Build history of the part. All positions in model axes, mm. A direction names the side the tool comes from. Round coordinates to 2 decimals unless told otherwise and drop trailing zeros. Loops run counter-clockwise (first coordinate to the right, second up) from the corner with the lowest first, then second, coordinate; pieces in that order, holes last. Notation, with made-up numbers: M -39,-31 L 2,-31 A34 ccw 2,1 Z; hole C -30.5,10.5 d10. An arc over 180 degrees is marked long. Use one line per item in the form item = value. Start each with the question number.
```python
from build123d import *

# Parameters (mm, degrees)
F1_DEPTH = 70
F2_T     = -1
F4_DEPTH = 4


with BuildPart() as f1:
    # F0 (on Top) → F1 (new body)
    with BuildSketch(Plane.XY):
        Polygon((50.477442, 204.086703), (-26.674857, 204.086703), (-79.522558, -15.913297), (-79.522558, -65.913297), (50.477442, -65.913297), align=None)
    extrude(amount=F1_DEPTH)

    # F2
    f2_openings = [f1.faces().sort_by_distance(p)[0] for p in [
        (-5.117094, 56.846235, 70),
    ]]
    offset(amount=F2_T, openings=f2_openings)

    # F3 (on face) → F4 (cut)
    with BuildSketch(Plane(origin=(-71.57003, 17.192325, 0), x_dir=(-0.233572, -0.972339, 0), z_dir=(-0.972339, 0.233572, 0))):
        Polygon((-165.007069, 17.787976), (-173.111157, 26.931221), (-184.3112, 22.049193), (-183.12912, 9.888689), (-171.19851, 7.255112), align=None)
    extrude(amount=-F4_DEPTH, mode=Mode.SUBTRACT)


solid = f1.part
```
Q1. Saw through at B-B (x = 32). Give the cut face in (y, z), and give its area (3 significant figures).
Q2. Saw through at A-A (z = 35). Give the cut face in (x, y).
Q3. Saw through at C-C (y = -39). Give the cut face in (x, z).
Q4. Tool access for faces 4 (the face through (12, 204.087, 35)), 5 (the face through (-15, -64.913, 35)): list every direction of +Z, -Z, +X, -X, +Y, -Y with a clear straight run to the whole face (end or side of a thin tool).
Q5. Wall check: probe 1 along Y at (x, z) = (-4, 44.5); probe 2 along X at (y, z) = (-27, 57.5); probe 3 along Z at (x, y) = (-33, 62.5). Give the ranges that are in metal, low to high.
Q6. Drop flat-ended pins along their axis: P1, Ø8, axis at x = -23.5, y = 99.5, coming from the -Z side; P2, Ø12, axis at y = 23.5, z = 50.5, coming from the -X side; P3, Ø8, axis at y = 172.5, z = 27.5, coming from the -X side; P4, Ø5, axis at x = 28.5, y = 170, coming from the +Z side. Give the stop position or say it passes through.
Q7. Pull direction X, two halves, no side cores. Call faces 1 (the face through (-15, -65.913, 35)), 2 (the face through (-51.836, 95.061, 35.017)), 3 (the face through (-79.523, -41, 35)): pulls with the +X half, pulls with the -X half, needs draft (parallel to the pull), parting line crosses it, or undercut.
Filled in:
q1.outline = M -65.91,0 L 204.09,0 L 204.09,70 L 203.09,70 L 203.09,1 L -64.91,1 L -64.91,70 L -65.91,70 Z
q1.area = 408 mm²
q2.outline = M -79.52,-65.91 L 50.48,-65.91 L 50.48,204.09 L -26.67,204.09 L -79.52,-15.91 Z; hole M -78.52,-64.91 L 49.48,-64.91 L 49.48,203.09 L -25.89,203.09 L -78.52,-16.03 Z
q3.outline = M -79.52,0 L 50.48,0 L 50.48,70 L 49.48,70 L 49.48,1 L -78.52,1 L -78.52,70 L -79.52,70 Z
q4.face_4 = +Z, -Z, +X, -X, +Y
q4.face_5 = +Z
q5.probe_1 = -65.91 to -64.91, 203.09 to 204.09
q5.probe_2 = -79.52 to -78.52, 49.48 to 50.48
q5.probe_3 = 0 to 1
q6.P1 = 0
q6.P2 = -71.5
q6.P3 = -35.22
q6.P4 = 1
q7.face_1 = needs draft
q7.face_2 = undercut
q7.face_3 = pulls with the -X half
